```python
from build123d import *

# Parameters (mm, degrees)
SKETCH1_R                  = 2
BOSS_EXTRUDE1_DEPTH        = 3
F_3_5_3_5_DIAMETER_HOLE1_D = 3.5
SKETCH4_W                  = 4
SKETCH4_H                  = 2
CUT_EXTRUDE1_DEPTH         = 110.813478226


with BuildPart() as part:
    # Sketch1 → Boss-Extrude1 (new body)
    with BuildSketch(Plane.XY):
        with BuildLine():
            Line((-82, 55), (82, 55))
            ThreePointArc((82, 55), (84.121320344, 54.121320344), (85, 52))
            Line((85, 52), (85, 41))
            ThreePointArc((85, 41), (86.464466094, 37.464466094), (90, 36))
            Line((90, 36), (92, 36))
            ThreePointArc((92, 36), (94.121320344, 35.121320344), (95, 33))
            Line((95, 33), (95, -33))
            ThreePointArc((95, -33), (94.121320344, -35.121320344), (92, -36))
            Line((92, -36), (90, -36))
            ThreePointArc((90, -36), (86.464466094, -37.464466094), (85, -41))
            Line((85, -41), (85, -52))
            ThreePointArc((85, -52), (84.121320344, -54.121320344), (82, -55))
            Line((82, -55), (-82, -55))
            ThreePointArc((-82, -55), (-84.121320344, -54.121320344), (-85, -52))
            Line((-85, -52), (-85, -41))
            ThreePointArc((-85, -41), (-86.464466094, -37.464466094), (-90, -36))
            Line((-90, -36), (-92, -36))
            ThreePointArc((-92, -36), (-94.121320344, -35.121320344), (-95, -33))
            Line((-95, -33), (-95, 33))
            ThreePointArc((-95, 33), (-94.121320344, 35.121320344), (-92, 36))
            Line((-92, 36), (-90, 36))
            ThreePointArc((-90, 36), (-86.464466094, 37.464466094), (-85, 41))
            Line((-85, 41), (-85, 52))
            ThreePointArc((-85, 52), (-84.121320344, 54.121320344), (-82, 55))
        make_face()
        with Locations((-80.5, 45)):
            Circle(SKETCH1_R, mode=Mode.SUBTRACT)
        with Locations((19.5, 45)):
            Circle(SKETCH1_R, mode=Mode.SUBTRACT)
        with Locations((80.5, 45)):
            Circle(SKETCH1_R, mode=Mode.SUBTRACT)
        with Locations((-80.5, -45)):
            Circle(SKETCH1_R, mode=Mode.SUBTRACT)
        with Locations((-87.5, 0)):
            Circle(SKETCH1_R, mode=Mode.SUBTRACT)
        with Locations((87.5, 0)):
            Circle(SKETCH1_R, mode=Mode.SUBTRACT)
        with Locations((19.5, -45)):
            Circle(SKETCH1_R, mode=Mode.SUBTRACT)
        with Locations((80.5, -45)):
            Circle(SKETCH1_R, mode=Mode.SUBTRACT)
    extrude(amount=BOSS_EXTRUDE1_DEPTH)

    # Ø3.5 (3.5) Diameter Hole1 (through all)
    with Locations(Plane.XY.offset(3)):
        with Locations((88, 7.7), (88, -17.7), (62.6, -17.7), (62.6, 7.7), (-73, 14), (-15, 14), (-15, -35), (-73, -35)):
            Hole(F_3_5_3_5_DIAMETER_HOLE1_D / 2)

    # Sketch4 → Cut-Extrude1 (cut, through all)
    with BuildSketch(Plane.XY.offset(3)):
        with Locations((-9.482801071, 33.175325002)):
            Rectangle(SKETCH4_W, SKETCH4_H)
        with Locations((-49.482801071, 33.175325002)):
            Rectangle(SKETCH4_W, SKETCH4_H)
        with Locations((-49.482801071, 29.175325002)):
            Rectangle(SKETCH4_W, SKETCH4_H)
        with Locations((-9.482801071, 29.175325002)):
            Rectangle(SKETCH4_W, SKETCH4_H)
        with Locations((30.517198929, 33.175325002)):
            Rectangle(SKETCH4_W, SKETCH4_H)
        with Locations((30.517198929, 29.175325002)):
            Rectangle(SKETCH4_W, SKETCH4_H)
        with Locations((30.517198929, 13.175325002)):
            Rectangle(SKETCH4_W, SKETCH4_H)
        with Locations((30.517198929, 9.175325002)):
            Rectangle(SKETCH4_W, SKETCH4_H)
        with Locations((30.517198929, -6.824674998)):
            Rectangle(SKETCH4_W, SKETCH4_H)
        with Locations((30.517198929, -10.824674998)):
            Rectangle(SKETCH4_W, SKETCH4_H)
        with Locations((30.517198929, -26.824674998)):
            Rectangle(SKETCH4_W, SKETCH4_H)
        with Locations((30.517198929, -30.824674998)):
            Rectangle(SKETCH4_W, SKETCH4_H)
    extrude(amount=-CUT_EXTRUDE1_DEPTH, mode=Mode.SUBTRACT)


solid = part.part
```
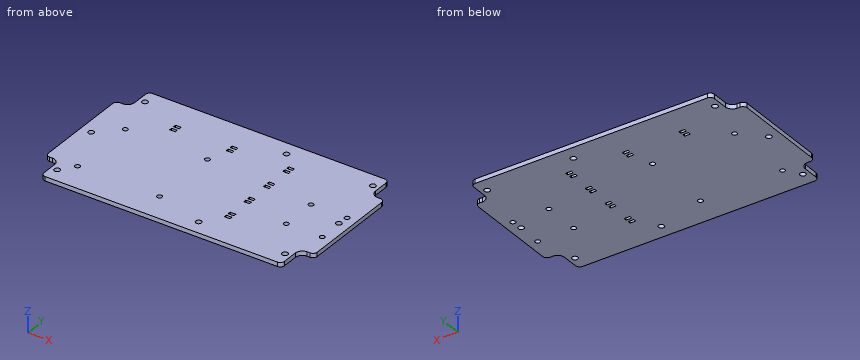
Verification items for the finished model (mm, model axes). Round coordinates to 2 decimals unless told otherwise and drop trailing zeros. Write each loop counter-clockwise with the first axis right and the second up, starting at its lowest first coordinate (ties: lowest second). Pieces come first, ordered by that corner, then holes.
1. Section check A-A on y = -45. Enter the section's corners in (x, z), plus the area to 3 significant figures.
2. Section check B-B on x = 19.5. Enter the section's corners in (y, z).
3. Scan lines: L1, parallel to Y at x = 62.6, z = 0.7; L2, parallel to Y at x = -50.5, z = 0.7; L3, parallel to Y at x = 87.5, z = 1.2. Record each from-to range of solid material in increasing order.
4. Section check C-C on z = 1.55. State how many separate pieces and enclosed holes the cut face has, plus the area to 3 significant figures.
5. Gauge pin test, flat ends, axial feed: P1, Ø0.9, axis at y = -49, z = 2, coming from the +X side; P2, Ø3, axis at x = -73, y = -35, coming from the -Z side. Record the tip position at first contact, or that the pin passes through.
Answer:
1. outline: (-85, 0) - (-82.5, 0) - (-82.5, 3) - (-85, 3) - close; (-78.5, 0) - (17.5, 0) - (17.5, 3) - (-78.5, 3) - close; (21.5, 0) - (78.5, 0) - (78.5, 3) - (21.5, 3) - close; (82.5, 0) - (85, 0) - (85, 3) - (82.5, 3) - close
1. area: 474 mm2
2. outline: (-55, 0) - (-47, 0) - (-47, 3) - (-55, 3) - close; (-43, 0) - (43, 0) - (43, 3) - (-43, 3) - close; (47, 0) - (55, 0) - (55, 3) - (47, 3) - close
3. L1: y = -55 to -19.45, -15.95 to 5.95, 9.45 to 55
3. L2: y = -55 to 28.18, 30.18 to 32.18, 34.18 to 55
3. L3: y = -36.67 to -19.38, -16.02 to -2, 2 to 6.02, 9.38 to 36.67
4. separate pieces: 1
4. enclosed holes: 28
4. area: 19,900 mm2
5. P1: stops at x = 85
5. P2: passes through
